from build123d import *

# Parameters (mm, degrees)
SWEEP_1_PROFILE_R = 0.6


with BuildPart() as part:
    # 扫描1: sweep along a path in 草图1
    with BuildLine(Plane.XY) as sweep_1_path:
        Line((-2, 3.464101615), (-0.433012702, 0.75))
        ThreePointArc((-0.433012702, 0.75), (0.116025404, 0.200961894), (0.866025404, 0))
        Line((0.866025404, 0), (3, 0))
        ThreePointArc((3, 0), (4.060660172, -0.439339828), (4.5, -1.5))
        Line((4.5, -1.5), (4.5, -38.5))
        ThreePointArc((4.5, -38.5), (4.939339828, -39.560660172), (6, -40))
        Line((6, -40), (11.5, -40))
    # 扫描1 profile (on start of the path) → 扫描1 (sweep)
    with BuildSketch(Plane(origin=(-2, 3.464101615, 0), x_dir=(-0.8660254037844379, -0.5000000000000013, 0), z_dir=(0.5000000000000013, -0.8660254037844379, 0))):
        Circle(SWEEP_1_PROFILE_R)
    sweep(path=sweep_1_path.line)


solid = part.part
Model file for the job. Use its own axes, mm. A direction names the side the tool comes from. Give positions to 0.01 mm unless a question says otherwise; leave off trailing zeros. Loops run counter-clockwise (first coordinate to the right, second up) from the corner with the lowest first, then second, coordinate; pieces in that order, holes last. Notation, with made-up numbers: (-22.75, -21) -> (33.25, -21) arc R30 ccw to (33.25, 16) -> close; hole circle Ø4 at (78.25, -17.75). An arc over 180 degrees is marked (long way). Use a Markdown table: item, result. Add a question column.
(1) Slice it at A-A on z = 0. List the corners of the cut face in (x, y).
(2) Slice it at C-C on y = -17. List the corners of the cut face in (x, z).
(3) Slice it at B-B on x = 10.75. List the corners of the cut face in (y, z).
(4) Wall check: line 1 along Y through (x, z) = (10.75, 0); line 2 along Y through (x, z) = (1.25, -0.1); line 3 along X through (y, z) = (-16.5, -0.1). Give the ranges that are in metal, low to high.
(5) Mould opens along Y. For faces 1 (the cylindrical face through (5.1, -20.3, 0)), 2 (the cylindrical face through (8.788, -40.554, 0.23)), 3 (the flat face through (-1.99, 3.47, -0.01)) say: +Y half, -Y half, draft (parallel to the pull), parting line (faces both ways), or undercut.
(6) Tool access for faces 4 (the flat face through (11.5, -40, 0)), 5 (the cylindrical face through (1.948, -0.323, -0.506)): list every direction of +Z, -Z, +X, -X, +Y, -Y with a clear straight run to the whole face (end or side of a thin tool).
Filled sheet:
| question | item | result |
|---|---|---|
| 1 | outline | (-2.52, 3.16) -> (-0.95, 0.45) arc R2.1 ccw to (0.87, -0.6) -> (3, -0.6) arc R0.9 cw to (3.9, -1.5) -> (3.9, -38.5) arc R2.1 ccw to (6, -40.6) -> (11.5, -40.6) -> (11.5, -39.4) -> (6, -39.4) arc R0.9 cw to (5.1, -38.5) -> (5.1, -1.5) arc R2.1 ccw to (3, 0.6) -> (0.87, 0.6) arc R0.9 cw to (0.09, 1.05) -> (-1.48, 3.76) -> close |
| 2 | outline | circle Ø1.2 at (4.5, 0) |
| 3 | outline | circle Ø1.2 at (-40, 0) |
| 4 | line 1 | -40.6 to -39.4 |
| 4 | line 2 | -0.59 to 0.59 |
| 4 | line 3 | 3.91 to 5.09 |
| 5 | face 1 | draft |
| 5 | face 2 | parting line |
| 5 | face 3 | +Y half |
| 6 | face 4 | +Z, -Z, +X, +Y, -Y |
| 6 | face 5 | none |
